Drawing for the job (mm, zero at the part's lowest x, y, z). Coordinates: 2 decimals unless noted, no trailing zeros. Order: outer loops, then holes, each group sorted by start corner. A loop starts at its lowest first (then second) coordinate and runs counter-clockwise, first axis right, second up. Notation, with made-up numbers: M 47.5,-3.5 L 100.5,-3.5 A20 ccw 100.5,19.5 Z; hole C -20.75,3.5 d3. An arc over 180 degrees is marked long. Write item = value, one per line. Start each with the question number.
Q1. Pin check, flat tip, straight feed: P1, Ø2, axis at y = 2.5, z = 56, coming from the -X side. Stop position of the tip, or through.
Q2. Band-saw the part on C-C on x = 36.5. Write the cut outline in (y, z).
Q3. Drill centre lines: probe 1 along Z at (x, y) = (17, 5.25); probe 2 along Z at (x, y) = (103.5, 2); probe 3 along X at (y, z) = (3.25, 66.5). Where is each one in solid material? Low to high.
Q4. Band-saw the part on D-D on y = 5. Write the cut outline in (x, z), plus the area to 3 significant figures.
Q5. Band-saw the part on A-A on x = 11.5. Write the cut outline in (y, z), plus the area to 3 significant figures.
Q6. Band-saw the part on B-B on z = 94. Write the cut outline in (x, y), plus the area to 3 significant figures.
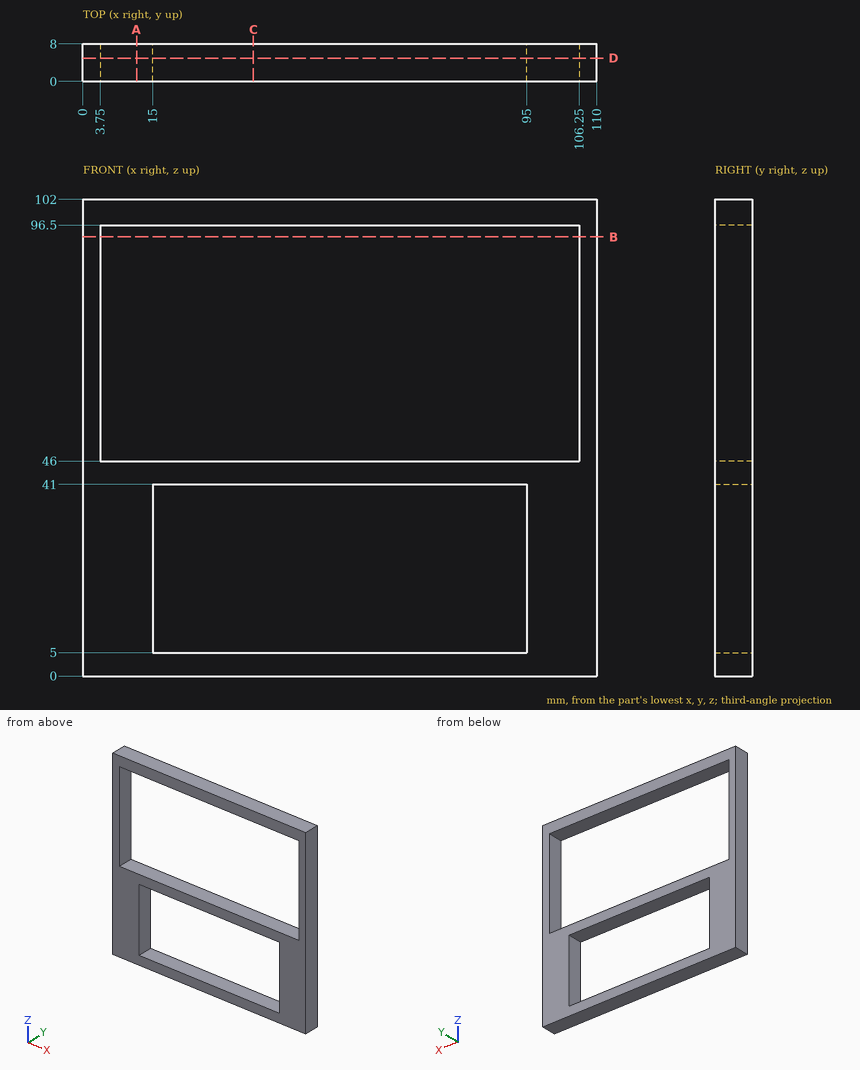
Recorded:
q1.P1 = 0
q2.outline = M 0,0 L 8,0 L 8,5 L 0,5 Z; M 0,41 L 8,41 L 8,46 L 0,46 Z; M 0,96.5 L 8,96.5 L 8,102 L 0,102 Z
q3.probe_1 = 0 to 5, 41 to 46, 96.5 to 102
q3.probe_2 = 0 to 46, 96.5 to 102
q3.probe_3 = 0 to 3.75, 106.25 to 110
q4.outline = M 0,0 L 110,0 L 110,102 L 0,102 Z; hole M 3.75,46 L 106.25,46 L 106.25,96.5 L 3.75,96.5 Z; hole M 15,5 L 95,5 L 95,41 L 15,41 Z
q4.area = 3,160 mm2
q5.outline = M 0,0 L 8,0 L 8,46 L 0,46 Z; M 0,96.5 L 8,96.5 L 8,102 L 0,102 Z
q5.area = 412 mm2
q6.outline = M 0,0 L 3.75,0 L 3.75,8 L 0,8 Z; M 106.25,0 L 110,0 L 110,8 L 106.25,8 Z
q6.area = 60.0 mm2
